Check sheet for the modelled part. Datum: model origin and axes. Units: mm. A direction names the side the tool comes from. Give positions to 0.01 mm unless a question says otherwise; leave off trailing zeros. Write each loop counter-clockwise with the first axis right and the second up, starting at its lowest first coordinate (ties: lowest second). Pieces come first, ordered by that corner, then holes. Notation, with made-up numbers: M 56.5,-3.5 L 114.5,-3.5 A11 ccw 114.5,9.5 Z; hole C -36.75,-11.75 d8. An arc over 180 degrees is marked long. Write item = value, one per line. Start each with the question number.
1) Scan lines: line 1 along Z through (x, y) = (0, 2.4); line 2 along Y through (x, z) = (4, -9); line 3 along Y through (x, z) = (-4, 7.75). Record each from-to range of solid material in increasing order. Write a range as [from, to].
2) Access from +Z, -Z, +X, -X, +Y, -Y to the whole of each face (thin tool, end or side, straight path). Record for faces 1 (the flat face through (2.2, 0, -8.4)), 2 (the flat face through (2, 5, 2)), 3 (the cylindrical face through (-4.57, 1.972, -7.167)).
3) Cross-section at B-B, the plane x = 0. Record the cut outline in (y, z), plus the area to 3 significant figures.
4) Cross-section at A-A, the plane z = 0. Record the cut outline in (x, y).
5) Cross-section at D-D, the plane x = 7.75. Record the cut outline in (y, z).
6) Mould release check, pull along Z, two halves, no side actions. Record for faces 4 (the cylindrical face through (-4.38, 1.48, 8.43)), 5 (the flat face through (-3, 6, 0)), 6 (the flat face through (9, 4, 0)): released by +Z, released by -Z, zero draft, split by the parting line, or undercut.
7) Go/stop test with a flat-tipped pin: pin 1 (6 mm diameter, centred on x = 0, z = 0, fed in from -Y). Record where the tip stops, or that it passes through.
8) Cross-section at C-C, the plane y = 2.55. Record the cut outline in (x, z), plus the area to 3 significant figures.
Autodesk Inventor part; units mm, degrees
ref_plane "YZ Plane" through (0, 0, 0) normal (1, 0, 0) x (0, 1, 0)
ref_plane "XZ Plane" through (0, 0, 0) normal (0, 1, 0) x (-1, 0, 0)
ref_plane "XY Plane" through (0, 0, 0) normal (0, 0, 1) x (1, 0, 0)
sketch "Sketch1" plane through (0, 0, 0) normal (0, 1, 0) x (-1, 0, 0)
  circle A0 centre (0, 0) radius 9.5
  dimension "d0" = 19
extrude "Extrusion1" add sketch "Sketch1" along normal blind 3
sketch "Sketch2" plane through (0, 3, 0) normal (0, 1, 0) x (1, 0, 0)
  circle A0 centre (0, 0) radius 11.5
  dimension "d3" = 23
extrude "Extrusion2" add sketch "Sketch2" along normal blind 3
shell "Shell1" thickness 1 removed faces 1 at (2.7119, 0, -0.7138)
sketch "Sketch3" plane through (0, 6, 0) normal (0, 1, 0) x (1, 0, 0)
  circle A0 centre (0, 0) radius 2.5
  dimension "d7" = 5
extrude "Extrusion3" cut sketch "Sketch3" against normal blind 3
properties part number "SwivelPartCap"
Reply:
q1.line_1 = [-9.5, -8.5], [8.5, 9.5]
q1.line_2 = [3, 4], [5, 6]
q1.line_3 = [0, 4], [5, 6]
q2.face_1 = +Z, -Z, +X, -X, -Y
q2.face_2 = none
q2.face_3 = -Y
q3.outline = M 0,-9.5 L 3,-9.5 L 3,-11.5 L 6,-11.5 L 6,-2.5 L 5,-2.5 L 5,-10.5 L 4,-10.5 L 4,-8.5 L 0,-8.5 Z; M 0,8.5 L 4,8.5 L 4,10.5 L 5,10.5 L 5,2.5 L 6,2.5 L 6,11.5 L 3,11.5 L 3,9.5 L 0,9.5 Z
q3.area = 32.0 mm2
q4.outline = M -11.5,3 L -9.5,3 L -9.5,0 L -8.5,0 L -8.5,4 L -10.5,4 L -10.5,5 L -2.5,5 L -2.5,6 L -11.5,6 Z; M 2.5,5 L 10.5,5 L 10.5,4 L 8.5,4 L 8.5,0 L 9.5,0 L 9.5,3 L 11.5,3 L 11.5,6 L 2.5,6 Z
q5.outline = M 0,-5.49 L 3,-5.49 L 3,-8.5 L 6,-8.5 L 6,8.5 L 3,8.5 L 3,5.49 L 0,5.49 L 0,3.49 L 4,3.49 L 4,7.08 L 5,7.08 L 5,-7.08 L 4,-7.08 L 4,-3.49 L 0,-3.49 Z
q6.face_4 = split by the parting line
q6.face_5 = zero draft
q6.face_6 = undercut
q7.pin_1 = 5
q8.outline = C 0,0 d19; hole C 0,0 d17
q8.area = 56.5 mm2
